from build123d import *

# Parameters (mm, degrees)
BOSS_EXTRUDE1_DEPTH = 30
SKETCH2_R           = 1.5
CUT_EXTRUDE1_DEPTH  = 40.819488185
SKETCH3_W           = 30
SKETCH3_H           = 12.5
BOSS_EXTRUDE2_DEPTH = 2.5


with BuildPart() as part:
    # Sketch1 → Boss-Extrude1 (new body)
    with BuildSketch(Plane.XY):
        with BuildLine():
            Line((16.007425743, 3.681930693), (23.007425743, 3.681930693))
            Line((23.007425743, 3.681930693), (23.007425743, -8.818069307))
            Line((23.007425743, -8.818069307), (-6.992574257, -8.818069307))
            Line((-6.992574257, -8.818069307), (-6.992574257, 3.681930693))
            Line((-6.992574257, 3.681930693), (0.007425743, 3.681930693))
            ThreePointArc((0.007425743, 3.681930693), (8.007425743, -4.318069307), (16.007425743, 3.681930693))
        make_face()
    extrude(amount=BOSS_EXTRUDE1_DEPTH)

    # Sketch2 → Cut-Extrude1 (cut, through all)
    with BuildSketch(Plane.XZ.offset(8.818069307)):
        with Locations(Location((-3.492574257, 3.5, 0), (0, 0, 270))):
            Circle(SKETCH2_R)
        with Locations(Location((-3.492574257, 26.5, 0), (0, 0, 270))):
            Circle(SKETCH2_R)
    extrude(amount=-CUT_EXTRUDE1_DEPTH, mode=Mode.SUBTRACT)

    # Sketch3 → Boss-Extrude2 (add)
    with BuildSketch(Plane.ZY.offset(6.992574257)):
        with Locations((15, -2.568069307)):
            Rectangle(SKETCH3_W, SKETCH3_H)
    extrude(amount=BOSS_EXTRUDE2_DEPTH)


solid = part.part
Read the model definition and answer for the solid it produces. Units are mm, in the model's axes. Give positions to 0.01 mm unless a question says otherwise; leave off trailing zeros. Write each loop counter-clockwise with the first axis right and the second up, starting at its lowest first coordinate (ties: lowest second). Pieces come first, ordered by that corner, then holes. Notation, with made-up numbers: (86, 46.5) - (116, 46.5) arc R30 ccw to (116, 72.5) - close; hole circle Ø3 at (43, -32.75). An arc over 180 degrees is marked (long way). Answer in a Markdown table with one row per item. Add a question column.
Item 1: Section D-D, the plane y = -3.25 is taken. Write down the section's boundary in (x, z), and give its area (3 significant figures).
Item 2: Section B-B, the plane y = 2 is taken. Write down the section's boundary in (x, z).
Item 3: Section C-C, the plane z = 16 is taken. Write down the section's boundary in (x, y).
Item 4: Find the intervals of material crossed by L1, parallel to X at y = -5.5, z = 26.5; L2, parallel to X at y = 1, z = 3.5; L3, parallel to X at y = 1.25, z = 3.5, in increasing order.
Item 5: Determine the mould class of faces 1 (the face through (7, -5, 0)), 2 (the face through (-3.04, -2.66, 2.07)), 3 (the face through (-9.493, -2, 15)) for opening direction X: pulls with the +X half, pulls with the -X half, needs draft (parallel to the pull), parting line crosses it, or undercut.
Item 6: Flat-ended cylindrical pins translate along their axes: P1, Ø6, axis at x = 4.5, z = 17, coming from the +Y side; P2, Ø6, axis at x = 10.5, z = 5.5, coming from the +Y side; P3, Ø2.5, axis at x = -3.49, z = 26.5, coming from the +Y side. Find the tip coordinate at first contact, or state that the pin passes through.
Item 7: Section A-A, the plane z = 3.5 is taken. Write down the section's boundary in (x, y).
Recorded:
| question | item | result |
|---|---|---|
| 1 | outline | (-9.49, 0) - (4.01, 0) - (4.01, 30) - (-9.49, 30) - close; (12, 0) - (23.01, 0) - (23.01, 30) - (12, 30) - close; hole circle Ø3 at (-3.49, 3.5); hole circle Ø3 at (-3.49, 26.5) |
| 1 | area | 721 mm2 |
| 2 | outline | (-9.49, 0) - (0.19, 0) - (0.19, 30) - (-9.49, 30) - close; (15.83, 0) - (23.01, 0) - (23.01, 30) - (15.83, 30) - close; hole circle Ø3 at (-3.49, 3.5); hole circle Ø3 at (-3.49, 26.5) |
| 3 | outline | (-9.49, -8.82) - (23.01, -8.82) - (23.01, 3.68) - (16.01, 3.68) arc R8 cw to (0.01, 3.68) - (-9.49, 3.68) - close |
| 4 | L1 | x = -9.49 to -4.99, -1.99 to 23.01 |
| 4 | L2 | x = -9.49 to -4.99, -1.99 to 0.47, 15.54 to 23.01 |
| 4 | L3 | x = -9.49 to -4.99, -1.99 to 0.39, 15.63 to 23.01 |
| 5 | face 1 | needs draft |
| 5 | face 2 | undercut |
| 5 | face 3 | pulls with the -X half |
| 6 | P1 | stops at y = -0.97 |
| 6 | P2 | stops at y = -2.13 |
| 6 | P3 | passes through |
| 7 | outline | (-9.49, -8.82) - (-4.99, -8.82) - (-4.99, 3.68) - (-9.49, 3.68) - close; (-1.99, -8.82) - (23.01, -8.82) - (23.01, 3.68) - (16.01, 3.68) arc R8 cw to (0.01, 3.68) - (-1.99, 3.68) - close |
